from build123d import *

# Parameters (mm, degrees)
BOSS_EXTRUDE1_DEPTH = 30
SKETCH2_R           = 3
CUT_EXTRUDE1_DEPTH  = 18
SKETCH3_R           = 1.75
CUT_EXTRUDE2_DEPTH  = 13
SKETCH4_R           = 1.5
CUT_EXTRUDE3_DEPTH  = 2


with BuildPart() as part:
    # Sketch1 → Boss-Extrude1 (new body)
    with BuildSketch(Plane(origin=(0, 0, 0), x_dir=(1, 0, 0), z_dir=(0, 1, 0))):
        with BuildLine():
            Line((0, 0), (15.5, 0))
            Line((15.5, 0), (15.5, 13.5))
            Line((15.5, 13.5), (11.75, 13.5))
            ThreePointArc((11.75, 13.5), (7.75, 14), (3.75, 13.5))
            Line((3.75, 13.5), (0, 13.5))
            Line((0, 13.5), (0, 0))
        make_face()
    extrude(amount=BOSS_EXTRUDE1_DEPTH)

    # Sketch2 → Cut-Extrude1 (cut)
    with BuildSketch(Plane(origin=(0, 30, 0), x_dir=(1, 0, 0), z_dir=(0, 1, 0))):
        with Locations((7.75, 6.75)):
            Circle(SKETCH2_R)
    extrude(amount=-CUT_EXTRUDE1_DEPTH, mode=Mode.SUBTRACT)

    # Sketch3 → Cut-Extrude2 (cut, through all)
    with BuildSketch(Plane(origin=(0, 12, 0), x_dir=(1, 0, 0), z_dir=(0, 1, 0))):
        with Locations((7.75, 6.75)):
            Circle(SKETCH3_R)
    extrude(amount=-CUT_EXTRUDE2_DEPTH, mode=Mode.SUBTRACT)

    # Sketch4 → Cut-Extrude3 (cut)
    with BuildSketch(Plane(origin=(15.5, 0, 0), x_dir=(0, 0, -1), z_dir=(1, 0, 0))):
        with Locations((6.75, 21.515)):
            Circle(SKETCH4_R)
        with Locations((6.75, 6.815)):
            Circle(SKETCH4_R)
    extrude(amount=-CUT_EXTRUDE3_DEPTH, mode=Mode.SUBTRACT)


solid = part.part
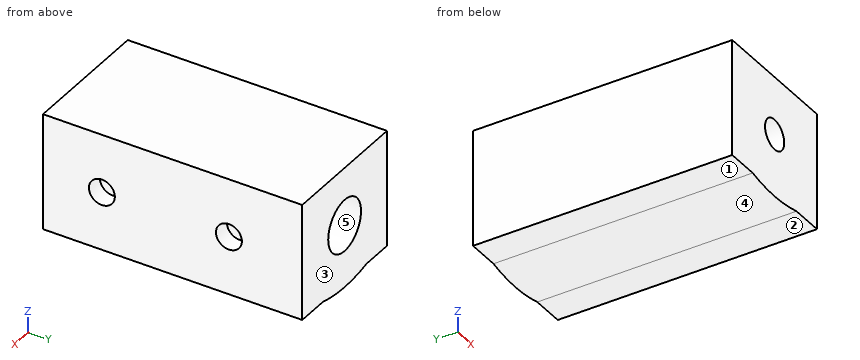
Can you work these out from the model? Positions are in its coordinate system, mm. Face numbers are marked on the shaded views. A direction names the side the tool comes from. Give positions to 0.01 mm unless a question says otherwise; leave off trailing zeros. Loops run counter-clockwise (first coordinate to the right, second up) from the corner with the lowest first, then second, coordinate; pieces in that order, holes last. Notation, with made-up numbers: (45, 35) - (71, 35) arc R23 cw to (71, 51) - close; hole circle Ø7 at (76, -17). An arc over 180 degrees is marked (long way). One line per item, written item: value.
(1) On a 3-axis mill with a long thin cutter (end or side, diameter ignored), from which of +Z, -Z, +X, -X, +Y, -Y can I reach the whole of each face in a straight line? I mean the marked faces 1, 2, 3, 4 and 5. Say none if no direction works.
Verdict:
face 1: -Z, -X, +Y, -Y
face 2: -Z, +X, +Y, -Y
face 3: +Z, -Z, +X, -X, +Y
face 4: -Z, +Y, -Y
face 5: +Y
(2) I need wall thicknesses on line 1 along Y through (x, z) = (15.05, -6.75) (3 decimals); line 2 along Z through (x, y) = (7.75, 5.75); line 3 along Z through (x, y) = (7.75, 24.75). Which ranges of each line are inside material? Lowest first, please.
Verdict:
line 1: 0 to 5.315, 8.315 to 20.015, 23.015 to 30
line 2: -14 to -8.5, -5 to 0
line 3: -14 to -9.75, -3.75 to 0
(3) If we section it at A-A, the plane z = -6.75: List the corners of the cut face in (x, y) for me (3 decimals), plus the area to 3 significant figures.
Verdict:
outline: (0, 0) - (6, 0) - (6, 12) - (4.75, 12) - (4.75, 30) - (0, 30) - close; (9.5, 0) - (15.5, 0) - (15.5, 5.315) - (13.5, 5.315) - (13.5, 8.315) - (15.5, 8.315) - (15.5, 20.015) - (13.5, 20.015) - (13.5, 23.015) - (15.5, 23.015) - (15.5, 30) - (10.75, 30) - (10.75, 12) - (9.5, 12) - close
area: 303 mm^2
(4) If we section it at B-B, the plane y = 15: List the corners of the cut face in (x, z) for me.
Verdict:
outline: (0, -13.5) - (3.75, -13.5) arc R16.25 ccw to (11.75, -13.5) - (15.5, -13.5) - (15.5, 0) - (0, 0) - close; hole circle Ø6 at (7.75, -6.75)
(5) If we section it at D-D, the plane y = 11: List the corners of the cut face in (x, z) for me.
Verdict:
outline: (0, -13.5) - (3.75, -13.5) arc R16.25 ccw to (11.75, -13.5) - (15.5, -13.5) - (15.5, 0) - (0, 0) - close; hole circle Ø3.5 at (7.75, -6.75)
(6) If we section it at C-C, the plane x = 7.75: List the corners of the cut face in (y, z) for me, plus the area to 3 significant figures.
Verdict:
outline: (0, -14) - (30, -14) - (30, -9.75) - (12, -9.75) - (12, -8.5) - (0, -8.5) - close; (0, -5) - (12, -5) - (12, -3.75) - (30, -3.75) - (30, 0) - (0, 0) - close
area: 270 mm^2
(7) I'm going to push flat-ended pins straight in: pin 1 (4 mm diameter, centred on x = 14, y = 14.5, fed in from -Z); pin 2 (3 mm diameter, centred on x = 8.5, z = -7.5, fed in from +Y); pin 3 (1.5 mm diameter, centred on y = 21, z = -7, fed in from +X). Where does each tip first touch, or does it pass through?
Verdict:
pin 1: z = -13.5
pin 2: y = 12
pin 3: x = 13.5
